from build123d import *

# Parameters (mm, degrees)
BOSS_EXTRUDE1_DEPTH = 60
CUT_EXTRUDE1_DEPTH  = 120


with BuildPart() as part:
    # Sketch1 → Boss-Extrude1 (new, symmetric)
    with BuildSketch(Plane(origin=(0, 0, 0), x_dir=(0, 0, -1), z_dir=(1, 0, 0))):
        with BuildLine():
            Line((12.25, 0), (-12.25, 0))
            ThreePointArc((-12.25, 0), (-13.133883476, 0.366116524), (-13.5, 1.25))
            Line((-13.5, 1.25), (-13.5, 5.25))
            ThreePointArc((-13.5, 5.25), (-13.866116524, 6.133883476), (-14.75, 6.5))
            Line((-14.75, 6.5), (-17.5, 6.5))
            Line((-17.5, 6.5), (-17.5, 7.5))
            Line((-17.5, 7.5), (-14.75, 7.5))
            ThreePointArc((-14.75, 7.5), (-13.159009742, 6.840990258), (-12.5, 5.25))
            Line((-12.5, 5.25), (-12.5, 1.25))
            ThreePointArc((-12.5, 1.25), (-12.426776695, 1.073223305), (-12.25, 1))
            Line((-12.25, 1), (12.25, 1))
            ThreePointArc((12.25, 1), (12.426776695, 1.073223305), (12.5, 1.25))
            Line((12.5, 1.25), (12.5, 5.25))
            ThreePointArc((12.5, 5.25), (13.159009742, 6.840990258), (14.75, 7.5))
            Line((14.75, 7.5), (17.5, 7.5))
            Line((17.5, 7.5), (17.5, 6.5))
            Line((17.5, 6.5), (14.75, 6.5))
            ThreePointArc((14.75, 6.5), (13.866116524, 6.133883476), (13.5, 5.25))
            Line((13.5, 5.25), (13.5, 1.25))
            ThreePointArc((13.5, 1.25), (13.133883476, 0.366116524), (12.25, 0))
        make_face()
    extrude(amount=BOSS_EXTRUDE1_DEPTH, both=True)

    # Sketch2 → Cut-Extrude1 (cut)
    with BuildSketch(Plane.XZ):
        with BuildLine():
            Line((-4.83, 3.17), (4.83, 3.17))
            ThreePointArc((4.83, 3.17), (8, 0), (4.83, -3.17))
            Line((4.83, -3.17), (-4.83, -3.17))
            ThreePointArc((-4.83, -3.17), (-8, 0), (-4.83, 3.17))
        make_face()
        with BuildLine():
            Line((18.17, -3.17), (27.83, -3.17))
            ThreePointArc((27.83, -3.17), (31, 0), (27.83, 3.17))
            Line((27.83, 3.17), (18.17, 3.17))
            ThreePointArc((18.17, 3.17), (15, 0), (18.17, -3.17))
        make_face()
        with BuildLine():
            Line((-27.83, -3.17), (-18.17, -3.17))
            ThreePointArc((-18.17, -3.17), (-15, 0), (-18.17, 3.17))
            Line((-18.17, 3.17), (-27.83, 3.17))
            ThreePointArc((-27.83, 3.17), (-31, 0), (-27.83, -3.17))
        make_face()
        with BuildLine():
            Line((-50.83, 3.17), (-41.17, 3.17))
            ThreePointArc((-41.17, 3.17), (-38, 0), (-41.17, -3.17))
            Line((-41.17, -3.17), (-50.83, -3.17))
            ThreePointArc((-50.83, -3.17), (-54, 0), (-50.83, 3.17))
        make_face()
        with BuildLine():
            Line((41.17, 3.17), (50.83, 3.17))
            ThreePointArc((50.83, 3.17), (54, 0), (50.83, -3.17))
            Line((50.83, -3.17), (41.17, -3.17))
            ThreePointArc((41.17, -3.17), (38, 0), (41.17, 3.17))
        make_face()
    extrude(amount=-CUT_EXTRUDE1_DEPTH, mode=Mode.SUBTRACT)


solid = part.part
Can you work these out from the model? Positions are in its coordinate system, mm. A direction names the side the tool comes from. Coordinates: 2 decimals unless noted, no trailing zeros. Write each loop counter-clockwise with the first axis right and the second up, starting at its lowest first coordinate (ties: lowest second). Pieces come first, ordered by that corner, then holes. Notation, with made-up numbers: M 32,-0.75 L 69,-0.75 A15 ccw 69,16.25 Z; hole C -21,-13 d2. An arc over 180 degrees is marked long. Use one line per item in the form item = value.
Q1. If we section it at C-C (z = 0): Write out the boundary of the cut face in (x, y), then the cut area to 3 significant figures.
Model answer:
outline = M -60,0 L -54,0 L -54,1 L -60,1 Z; M -38,0 L -31,0 L -31,1 L -38,1 Z; M -15,0 L -8,0 L -8,1 L -15,1 Z; M 8,0 L 15,0 L 15,1 L 8,1 Z; M 31,0 L 38,0 L 38,1 L 31,1 Z; M 54,0 L 60,0 L 60,1 L 54,1 Z
area = 40.0 mm^2
Q2. I need wall thicknesses on line 1 along Z through (x, y) = (24, 2.75); line 2 along Y through (x, z) = (54, -14.5); line 3 along Y through (x, z) = (-32, 2). Which ranges of each line are inside material? Lowest first, please. Write a range as from..to.
Model answer:
line_1 = -13.5..-12.5, 12.5..13.5
line_2 = 6.47..7.49
line_3 = 0..1
Q3. If we section it at B-B (x = 22): Write out the boundary of the cut face in (y, z).
Model answer:
outline = M 0,-12.25 A1.25 ccw 1.25,-13.5 L 5.25,-13.5 A1.25 cw 6.5,-14.75 L 6.5,-17.5 L 7.5,-17.5 L 7.5,-14.75 A2.25 ccw 5.25,-12.5 L 1.25,-12.5 A0.25 cw 1,-12.25 L 1,-3.17 L 0,-3.17 Z; M 0,3.17 L 1,3.17 L 1,12.25 A0.25 cw 1.25,12.5 L 5.25,12.5 A2.25 ccw 7.5,14.75 L 7.5,17.5 L 6.5,17.5 L 6.5,14.75 A1.25 cw 5.25,13.5 L 1.25,13.5 A1.25 ccw 0,12.25 Z
Q4. For faces 1 (the flat face through (1, 6.5, 16)), 2 (the cylindrical face through (-38, 0.5, 0.1)), 3 (the flat face through (1, 6.5, -16)), which set-ups out of +Z, -Z, +X, -X, +Y, -Y let a thin tool reach every point of the face, with its end or its side?
Model answer:
face_1 = +Z, +X, -X, -Y
face_2 = +Y, -Y
face_3 = -Z, +X, -X, -Y
Q5. If we section it at A-A (y = 4): Write out the boundary of the cut face in (x, z).
Model answer:
outline = M -60,-13.5 L 60,-13.5 L 60,-12.5 L -60,-12.5 Z; M -60,12.5 L 60,12.5 L 60,13.5 L -60,13.5 Z
Q6. If we section it at D-D (x = 34.5): Write out the boundary of the cut face in (y, z), then the cut area to 3 significant figures.
Model answer:
outline = M 0,-12.25 A1.25 ccw 1.25,-13.5 L 5.25,-13.5 A1.25 cw 6.5,-14.75 L 6.5,-17.5 L 7.5,-17.5 L 7.5,-14.75 A2.25 ccw 5.25,-12.5 L 1.25,-12.5 A0.25 cw 1,-12.25 L 1,12.25 A0.25 cw 1.25,12.5 L 5.25,12.5 A2.25 ccw 7.5,14.75 L 7.5,17.5 L 6.5,17.5 L 6.5,14.75 A1.25 cw 5.25,13.5 L 1.25,13.5 A1.25 ccw 0,12.25 Z
area = 45.9 mm^2
Q7. For P1, Ø0.5, axis at x = -45.5, y = 0.5, coming from the -Z side; P2, Ø10, axis at x = -34.5, z = -3.5, coming from the -Y side; P3, Ø1.2, axis at x = 17.5, y = 2.5, coming from the +Z side; P4, Ø0.8, axis at x = -43.5, y = 0.5, coming from the +Z side, each with a flat end and sliding along its axis, tell me the tip position at first contact or that it passes through.
Model answer:
P1 = -13.4
P2 = 0
P3 = 13.5
P4 = 13.45
Q8. We'd pull the mould along X, two halves only. Please class faces 4 (the flat face through (-60, 0.4, -0.1)), 5 (the cylindrical face through (-54, 0.5, -0.1)), 6 (the cylindrical face through (0.84, 6.82, -13.14)): +X half, -X half, draft (parallel to the pull), parting line (faces both ways), or undercut.
Model answer:
face_4 = -X half
face_5 = undercut
face_6 = draft
